Autodesk Fusion 360 part; units mm, degrees
sketch "Sketch1" plane through (0, 0, 0) normal (0, 0, 1) x (1, 0, 0)
  line L0 (54.2564, 77.5) -> (83.7564, 77.5)
  line L1 (83.7564, 77.5) -> (83.7564, 47.5)
  line L2 (83.7564, 47.5) -> (54.2564, 47.5)
  line L3 (54.2564, 47.5) -> (54.2564, 77.5)
  line L4 (83.7564, 77.5) -> (38.7564, 77.5)
  line L5 (38.7564, 77.5) -> (38.7564, 89.5)
  line L6 (38.7564, 89.5) -> (83.7564, 89.5)
  line L7 (83.7564, 89.5) -> (83.7564, 77.5)
  dimension "d3" = 29.5
  dimension "d4" = 30
  dimension "d5" = 12
  dimension "d6" = 45
extrude "Extrude1" add sketch "Sketch1" along normal blind 4
fillet "Fillet1" radius 17 1 edges at (83.7564, 89.5, 2)
CAD build for the part. Positions are in the model's coordinates, mm. A direction names the side the tool comes from. Coordinates: 2 decimals unless noted, no trailing zeros. Write each loop counter-clockwise with the first axis right and the second up, starting at its lowest first coordinate (ties: lowest second). Pieces come first, ordered by that corner, then holes.
(1) Cut at C-C, the plane x = 42. List the corners of the cut face in (y, z).
(2) Flat gauge pins, fed straight in: pin 1 (5 mm diameter, centred on x = 72.5, y = 52, fed in from -Z); pin 2 (6 mm diameter, centred on x = 51, y = 62, fed in from -Z); pin 3 (1.2 mm diameter, centred on x = 49, z = 2.5, fed in from -Y). Where does each tip first touch, or does it go through?
(3) Drill centre lines: probe 1 along Y at (x, z) = (51.5, 3.6); probe 2 along X at (y, z) = (54, 0.8); probe 3 along Y at (x, z) = (81, 0.6). Where is each one in solid material? Low to high.
(4) 3-axis set-ups, long thin cutter, end or side, ignore diameter. For faces 1 (the face through (83.756, 60, 2)), 2 (the face through (54.256, 62, 2)): which of +Z, -Z, +X, -X, +Y, -Y reach the whole face in a straight line?
(5) Cut at B-B, the plane y = 68. List the corners of the cut face in (x, z).
(6) Cut at A-A, the plane z = 3. List the corners of the cut face in (x, y).
Geometry says:
1. outline: (77.5, 0) - (89.5, 0) - (89.5, 4) - (77.5, 4) - close
2. pin 1: stops at z = 0
2. pin 2: passes through
2. pin 3: stops at y = 77.5
3. probe 1: y = 77.5 to 89.5
3. probe 2: x = 54.26 to 83.76
3. probe 3: y = 47.5 to 81.78
4. face 1: +Z, -Z, +X, +Y, -Y
4. face 2: +Z, -Z, -X, -Y
5. outline: (54.26, 0) - (83.76, 0) - (83.76, 4) - (54.26, 4) - close
6. outline: (38.76, 77.5) - (54.26, 77.5) - (54.26, 47.5) - (83.76, 47.5) - (83.76, 72.5) arc R17 ccw to (66.76, 89.5) - (38.76, 89.5) - close
